Autodesk Fusion 360 part; units mm, degrees
sketch "Sketch1" plane through (0, 0, 0) normal (0, 0, 1) x (1, 0, 0)
  circle A0 centre (0, 0) radius 5.75
  circle A1 centre (0, 0) radius 100.75
  circle A2 centre (0, 0) radius 3.975
  circle A3 centre (0, 0) radius 102.25
  line L0 (-25, -25) -> (25, -25)
  line L1 (25, -25) -> (25, 25)
  line L2 (25, 25) -> (-25, 25)
  line L3 (-25, 25) -> (-25, -25)
  line L4 (-25, -25) -> (25, 25) construction
  line L5 (25, -25) -> (-25, 25) construction
  circle A4 centre (25, -25) radius 3.5
  circle A5 centre (-25, -25) radius 3.5
  circle A6 centre (25, 25) radius 3.5
  circle A7 centre (-25, 25) radius 3.5
  circle A8 centre (-25, -25) radius 1.75
  circle A9 centre (-25, 25) radius 1.75
  circle A10 centre (25, 25) radius 1.75
  circle A11 centre (25, -25) radius 1.75
  dimension "d1" = 11.5
  dimension "d2" = 201.5
  dimension "d3" = 7.95
  dimension "d11" = 204.5
  dimension "d24" = 50
  dimension "d25" = 50
  dimension "d26" = 7
  dimension "d27" = 7
  dimension "d28" = 7
  dimension "d29" = 7
  dimension "d30" = 3.5
  dimension "d31" = 3.5
  dimension "d32" = 3.5
  dimension "d33" = 3.5
extrude "Extrude1" add sketch "Sketch1" along normal blind 6.5 contours A2
extrude "Extrude2" add sketch "Sketch1" against normal blind 3 contours A0 | A2
extrude "Extrude3" add sketch "Sketch1" against normal blind 3 from surface at -3 contours A0 | A1 | A2 | L0 L3 A8 | L0 L3 A8 | L0 L3 A5 A8 | L0 L3 A5 A8 | L0 L1 L2 L3 A4 A5 A6 A7 | L0 L1 A4 A11 | L0 L1 A4 A11 | L2 L3 A7 A9 | L2 L3 A7 A9 | L0 L1 A11 | L0 L1 A11 | L2 L3 A9 | L2 L3 A9 | L1 L2 A6 A10 | L1 L2 A6 A10 | L1 L2 A10 | L1 L2 A10
extrude "Extrude4" add sketch "Sketch1" along normal blind 68 from surface at -6 contours A3
chamfer "Chamfer1" distance 1 angle 45 1 edges at (-3.706, -1.4374, 6.5)
chamfer "Chamfer2" distance 0.5 angle 45 2 edges at (-95.3305, -36.9752, 62) (-93.932, 36.4328, 62)
chamfer "Chamfer3" distance 1 angle 45 1 edges at (-95.3305, -36.9752, -6)
extrude "Extrude6" cut sketch "Sketch1" against normal blind 15 contours L0 L3 A8 | L0 L3 A8 | L0 L1 A11 | L0 L1 A11 | L2 L3 A9 | L2 L3 A9 | L1 L2 A10 | L1 L2 A10
extrude "Extrude7" cut sketch "Sketch1" against normal blind 5 contours L0 L3 A5 A8 | L0 L3 A5 A8 | L0 L1 A4 A11 | L0 L1 A4 A11 | L2 L3 A7 A9 | L2 L3 A7 A9 | L1 L2 A6 A10 | L1 L2 A6 A10
extrude "Extrude9" cut sketch "Sketch1" along normal blind 45 from surface at 30 contours A3
chamfer "Chamfer4" distance 0.5 angle 45 2 edges at (-93.932, -36.4328, 30) (-95.3305, 36.9752, 30)
Read the model definition and answer for the solid it produces. Units are mm, in the model's axes. Round coordinates to 2 decimals unless told otherwise and drop trailing zeros. Order: outer loops, then holes, each group sorted by start corner. A loop starts at its lowest first (then second) coordinate and runs counter-clockwise, first axis right, second up. Notation, with made-up numbers: (-15.75, 15) - (34.25, 15) arc R26 ccw to (34.25, 50) - close; hole circle Ø10 at (-23.5, -4.5). An arc over 180 degrees is marked (long way). Use one line per item in the form item = value. Start each with the question number.
(1) Flat-ended cylindrical pins translate along their axes: pin 1 Ø3.5 at (x, y) = (-25.5, -26.5) entering from +Z; pin 2 Ø8 at (x, y) = (25, -25) entering from +Z; pin 3 Ø6.5 at (x, y) = (-0.5, -0.5) entering from +Z; pin 4 Ø3 at (x, y) = (25, 25) entering from -Z. Find the tip coordinate at first contact, or state that the pin passes through.
(2) The part is cut by section C-C (z = 22). Give the vertices of the cut face in (x, y).
(3) Find the intervals of material crossed by line 1 along Y through (x, z) = (25, -3.45); line 2 along Y through (x, z) = (25, -5.25); line 3 along Z through (x, y) = (-66.5, 47), in increasing order. Write a range as from..to.
(4) The part is cut by section A-A (x = 0). Give the vertices of the cut face in (y, z) (3 decimals), then the cut area to 3 significant figures.
(5) Determine the mould class of faces 1 (the face through (-23.12, -22.05, -3.99)), 2 (the face through (21, 1, -3)), 3 (the face through (-22.166, 99.819, 12.009)), 4 (the face through (-1, 1, -6)) for opening direction X: +X half, -X half, draft (parallel to the pull), parting line (faces both ways), or undercut.
Checked values:
q1.pin_1 = -5
q1.pin_2 = -3
q1.pin_3 = 6.5
q1.pin_4 = through
q2.outline = circle Ø204.5 at (0, 0); hole circle Ø201.5 at (0, 0)
q3.line_1 = -99.15..-28.5, -21.5..21.5, 28.5..99.15
q3.line_2 = -98.89..-26.75, -23.25..23.25, 26.75..98.89
q3.line_3 = -6..-3
q4.outline = (-102.25, -5) - (-101.25, -6) - (101.25, -6) - (102.25, -5) - (102.25, 29.5) - (101.75, 30) - (101.25, 30) - (100.75, 29.5) - (100.75, -3) - (5.75, -3) - (5.75, 0) - (3.975, 0) - (3.975, 5.5) - (2.975, 6.5) - (-2.975, 6.5) - (-3.975, 5.5) - (-3.975, 0) - (-5.75, 0) - (-5.75, -3) - (-100.75, -3) - (-100.75, 29.5) - (-101.25, 30) - (-101.75, 30) - (-102.25, 29.5) - close
q4.area = 796 mm^2
q5.face_1 = undercut
q5.face_2 = undercut
q5.face_3 = parting line
q5.face_4 = draft
